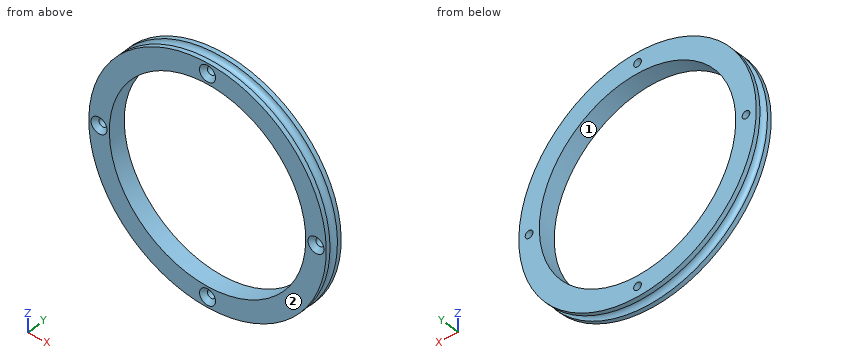
from build123d import *

# Parameters (mm, degrees)
CSK_FOR_M4_COUNTERSUNK_FLAT_HEAD_SCREW1_D           = 4.5
CSK_FOR_M4_COUNTERSUNK_FLAT_HEAD_SCREW1_CSINK_D     = 9.4
CSK_FOR_M4_COUNTERSUNK_FLAT_HEAD_SCREW1_CSINK_ANGLE = 90
CIRPATTERN1_COUNT                                   = 4


with BuildPart() as part:
    # Sketch1 → Revolve1 (revolve)
    with BuildSketch(Plane.XY, mode=Mode.PRIVATE) as revolve1_sk:
        with BuildLine():
            Line((-57.5, 5), (-57.5, -5))
            Line((-57.5, -5), (-69.5, -5))
            Line((-69.5, -5), (-69.5, -2.5))
            ThreePointArc((-69.5, -2.5), (-67, 0), (-69.5, 2.5))
            Line((-69.5, 2.5), (-69.5, 5))
            Line((-69.5, 5), (-57.5, 5))
        make_face()
    revolve(revolve1_sk.sketch.rotate(Axis((0, -5.61, 0), (0, 1, 0)), 270), axis=Axis((0, -5.61, 0), (0, 1, 0)))

    # CSK for M4 Countersunk Flat Head Screw1 (through all)
    with Locations(Plane(origin=(0, -5, 0), x_dir=(-1, 0, 0), z_dir=(0, -1, 0))):
        with Locations((63.5, 0)):
            csk_for_m4_countersunk_flat_head_screw1 = CounterSinkHole(CSK_FOR_M4_COUNTERSUNK_FLAT_HEAD_SCREW1_D / 2, CSK_FOR_M4_COUNTERSUNK_FLAT_HEAD_SCREW1_CSINK_D / 2, counter_sink_angle=CSK_FOR_M4_COUNTERSUNK_FLAT_HEAD_SCREW1_CSINK_ANGLE)

    # CirPattern1: CSK for M4 Countersunk Flat Head Screw1 ×4 about axis
    cirpattern1_axis = Axis((0, 0, 0), (0, 1, 0))
    for i in range(1, CIRPATTERN1_COUNT):
        add(csk_for_m4_countersunk_flat_head_screw1.rotate(cirpattern1_axis, i * 360 / CIRPATTERN1_COUNT), mode=Mode.SUBTRACT)


solid = part.part
For this review, take the finished solid that the model builds, in its own axes (mm). Face numbers are marked on the shaded views. Give positions to 0.01 mm unless a question says otherwise; leave off trailing zeros. Loops run counter-clockwise (first coordinate to the right, second up) from the corner with the lowest first, then second, coordinate; pieces in that order, holes last. Notation, with made-up numbers: M 37.25,69.25 L 48.25,69.25 A20 cw 48.25,108.25 Z; hole C -25.75,30.25 d7. An arc over 180 degrees is marked long. Put each result on its own line as item: value. Start each with the question number.
(1) Wall thickness on L1, parallel to Z at x = -5, y = 4.5; L2, parallel to X at y = 1.75, z = -45.5; L3, parallel to X at y = 0.75, z = 35.5: over which ranges is each line inside the solid? List them lowest first.
(2) Add section A-A, the plane z = 0. Write out the cut boundary in (x, y).
(3) Add section B-B, the plane y = 0. Write out the cut boundary in (x, z), then the cut area to 3 significant figures.
(4) The part is to be moulded in two halves that separate along X. For the marked faces 1 and 2, say which applies: +X half, -X half, draft (parallel to the pull), parting line (faces both ways), or undercut.
(5) Add section C-C, the plane x = 0. Write out the cut boundary in (y, z).
(6) For pin 1 (3 mm diameter, centred on x = -36, y = 1.5, fed in from +Z); pin 2 (6 mm diameter, centred on x = 0, z = -63.5, fed in from -Y); pin 3 (12 mm diameter, centred on x = 10, z = 51, fed in from +Y); pin 4 (5 mm diameter, centred on x = -25.5, y = 2.5, fed in from +Z), all flat-tipped, find the tip position at first contact; note any pin that passes through.
Result:
1. L1: z = -69.32 to -57.28, 57.28 to 69.32
1. L2: x = -50.15 to -35.16, 35.16 to 50.15
1. L3: x = -56.96 to -45.23, 45.23 to 56.96
2. outline: M -69.5,-5 L -68.2,-5 L -65.75,-2.55 L -65.75,5 L -69.5,5 L -69.5,2.5 A2.5 cw -69.5,-2.5 Z; M -61.25,-2.55 L -58.8,-5 L -57.5,-5 L -57.5,5 L -61.25,5 Z; M 57.5,-5 L 58.8,-5 L 61.25,-2.55 L 61.25,5 L 57.5,5 Z; M 65.75,-2.55 L 68.2,-5 L 69.5,-5 L 69.5,-2.5 A2.5 cw 69.5,2.5 L 69.5,5 L 65.75,5 Z
3. outline: C 0,0 d134; hole C -63.5,0 d4.5; hole C 0,0 d115; hole C 0,-63.5 d4.5; hole C 0,63.5 d4.5; hole C 63.5,0 d4.5
3. area: 3,650 mm^2
4. face 1: undercut
4. face 2: draft
5. outline: M -5,-69.5 L -2.5,-69.5 A2.5 cw 2.5,-69.5 L 5,-69.5 L 5,-65.75 L -2.55,-65.75 L -5,-68.2 Z; M -5,-58.8 L -2.55,-61.25 L 5,-61.25 L 5,-57.5 L -5,-57.5 Z; M -5,57.5 L 5,57.5 L 5,61.25 L -2.55,61.25 L -5,58.8 Z; M -5,68.2 L -2.55,65.75 L 5,65.75 L 5,69.5 L 2.5,69.5 A2.5 cw -2.5,69.5 L -5,69.5 Z
6. pin 1: stops at z = 60.11
6. pin 2: stops at y = -3.3
6. pin 3: stops at y = 5
6. pin 4: stops at z = 65.58
